Source: CAD feature listing. Evaluate the final solid. Frame: model axes, mm. Round coordinates to 2 decimals unless told otherwise and drop trailing zeros. Write each loop counter-clockwise with the first axis right and the second up, starting at its lowest first coordinate (ties: lowest second). Pieces come first, ordered by that corner, then holes. Notation, with made-up numbers: M -2,59 L 38,59 A24 ccw 38,87 Z; hole C -39.5,55 d1. An arc over 180 degrees is marked long. Answer in a Markdown table with one row per item.
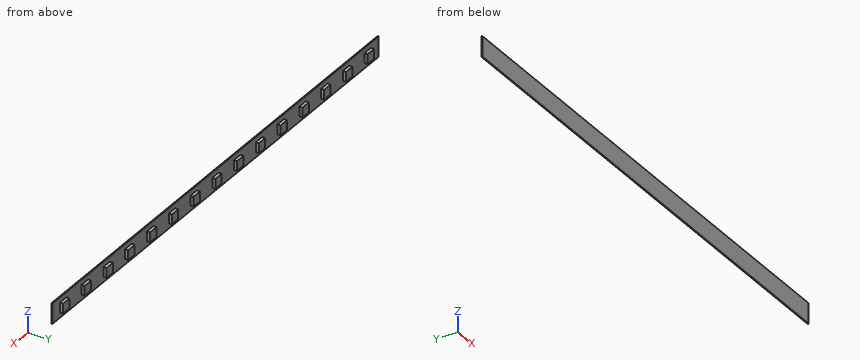
from build123d import *

# Parameters (mm, degrees)
SKETCH1_W           = 4.92
SKETCH1_H           = 4.92
BOSS_EXTRUDE1_DEPTH = 2
LPATTERN1_COUNT     = 15
LPATTERN1_PITCH     = 16.63
SKETCH2_W           = 249.45
SKETCH2_H           = 10.1
BOSS_EXTRUDE2_DEPTH = 0.5


with BuildPart() as part:
    # Sketch1 → Boss-Extrude1 (new body)
    with BuildSketch(Plane(origin=(0, 0, 0), x_dir=(1, 0, 0), z_dir=(0, 1, 0))):
        Rectangle(SKETCH1_W, SKETCH1_H)
    extrude(amount=BOSS_EXTRUDE1_DEPTH)


with BuildPart() as lpattern1_1:
    # LPattern1: pattern copy
    add(part.part.moved(Location(Vector(1, 0, 0) * (1 * LPATTERN1_PITCH))))


with BuildPart() as lpattern1_2:
    # LPattern1: pattern copy
    add(part.part.moved(Location(Vector(1, 0, 0) * (2 * LPATTERN1_PITCH))))


with BuildPart() as lpattern1_3:
    # LPattern1: pattern copy
    add(part.part.moved(Location(Vector(1, 0, 0) * (3 * LPATTERN1_PITCH))))


with BuildPart() as lpattern1_4:
    # LPattern1: pattern copy
    add(part.part.moved(Location(Vector(1, 0, 0) * (4 * LPATTERN1_PITCH))))


with BuildPart() as lpattern1_5:
    # LPattern1: pattern copy
    add(part.part.moved(Location(Vector(1, 0, 0) * (5 * LPATTERN1_PITCH))))


with BuildPart() as lpattern1_6:
    # LPattern1: pattern copy
    add(part.part.moved(Location(Vector(1, 0, 0) * (6 * LPATTERN1_PITCH))))


with BuildPart() as lpattern1_7:
    # LPattern1: pattern copy
    add(part.part.moved(Location(Vector(1, 0, 0) * (7 * LPATTERN1_PITCH))))


with BuildPart() as lpattern1_8:
    # LPattern1: pattern copy
    add(part.part.moved(Location(Vector(1, 0, 0) * (8 * LPATTERN1_PITCH))))


with BuildPart() as lpattern1_9:
    # LPattern1: pattern copy
    add(part.part.moved(Location(Vector(1, 0, 0) * (9 * LPATTERN1_PITCH))))


with BuildPart() as lpattern1_10:
    # LPattern1: pattern copy
    add(part.part.moved(Location(Vector(1, 0, 0) * (10 * LPATTERN1_PITCH))))


with BuildPart() as lpattern1_11:
    # LPattern1: pattern copy
    add(part.part.moved(Location(Vector(1, 0, 0) * (11 * LPATTERN1_PITCH))))


with BuildPart() as lpattern1_12:
    # LPattern1: pattern copy
    add(part.part.moved(Location(Vector(1, 0, 0) * (12 * LPATTERN1_PITCH))))


with BuildPart() as lpattern1_13:
    # LPattern1: pattern copy
    add(part.part.moved(Location(Vector(1, 0, 0) * (13 * LPATTERN1_PITCH))))


with BuildPart() as lpattern1_14:
    # LPattern1: pattern copy
    add(part.part.moved(Location(Vector(1, 0, 0) * (14 * LPATTERN1_PITCH))))


with BuildPart() as part_1:
    add(part.part)

    add(lpattern1_1.part)  # Boss-Extrude2 merges LPattern1_1

    add(lpattern1_2.part)  # Boss-Extrude2 merges LPattern1_2

    add(lpattern1_3.part)  # Boss-Extrude2 merges LPattern1_3

    add(lpattern1_4.part)  # Boss-Extrude2 merges LPattern1_4

    add(lpattern1_5.part)  # Boss-Extrude2 merges LPattern1_5

    add(lpattern1_6.part)  # Boss-Extrude2 merges LPattern1_6

    add(lpattern1_7.part)  # Boss-Extrude2 merges LPattern1_7

    add(lpattern1_8.part)  # Boss-Extrude2 merges LPattern1_8

    add(lpattern1_9.part)  # Boss-Extrude2 merges LPattern1_9

    add(lpattern1_10.part)  # Boss-Extrude2 merges LPattern1_10

    add(lpattern1_11.part)  # Boss-Extrude2 merges LPattern1_11

    add(lpattern1_12.part)  # Boss-Extrude2 merges LPattern1_12

    add(lpattern1_13.part)  # Boss-Extrude2 merges LPattern1_13

    add(lpattern1_14.part)  # Boss-Extrude2 merges LPattern1_14
    # Sketch2 → Boss-Extrude2 (add)
    with BuildSketch(Plane(origin=(0, 0, 0), x_dir=(1, 0, 0), z_dir=(0, 1, 0))):
        with Locations((116.41, 0)):
            Rectangle(SKETCH2_W, SKETCH2_H)
    extrude(amount=BOSS_EXTRUDE2_DEPTH)


solid = part_1.part
Q1. Section B-B (y = 1.15). State how many separate pieces and enclosed holes the cut face has, and give its area (3 significant figures).
Solutions:
| item | result |
|---|---|
| separate pieces | 15 |
| enclosed holes | 0 |
| area | 363 mm2 |
Q2. Section C-C (x = 76.5). Return loops of the section in (y, z).
Solutions:
| item | result |
|---|---|
| outline | M 0,-5.05 L 0.5,-5.05 L 0.5,5.05 L 0,5.05 Z |
Q3. Material intervals for probe 1 along Y at (x, z) = (125, -1.25); probe 2 along Z at (x, y) = (116, 1.8), sorted ascending.
Solutions:
| item | result |
|---|---|
| probe 1 | y = 0 to 0.5 |
| probe 2 | z = -2.46 to 2.46 |
Q4. Section A-A (x = 200). Return loops of the section in (y, z), and give its area (3 significant figures).
Solutions:
| item | result |
|---|---|
| outline | M 0,-5.05 L 0.5,-5.05 L 0.5,-2.46 L 2,-2.46 L 2,2.46 L 0.5,2.46 L 0.5,5.05 L 0,5.05 Z |
| area | 12.4 mm2 |
Q5. Contact query for flat-ended pins moving along their axis: pin 1 Ø0.8 at (x, y) = (148.5, 1) entering from +Z; pin 2 Ø0.8 at (y, z) = (1, 0) entering from -X; pin 3 Ø0.8 at (y, z) = (1.5, 0) entering from +X. Output: stop coordinate, or through.
Solutions:
| item | result |
|---|---|
| pin 1 | stops at z = 2.46 |
| pin 2 | stops at x = -2.46 |
| pin 3 | stops at x = 235.28 |
